Input: dimensioned drawing with shaded views. Units: mm. Origin: part minimum x, y, z. A direction names the side the tool comes from. Round coordinates to 2 decimals unless told otherwise and drop trailing zeros. Order: outer loops, then holes, each group sorted by start corner. A loop starts at its lowest first (then second) coordinate and runs counter-clockwise, first axis right, second up. Notation, with made-up numbers: M -30.75,72 L -9.75,72 A22 cw -9.75,101 Z; hole C -30.5,-12.5 d1. An arc over 180 degrees is marked long. Answer as CSV lines item,"result". Start each with the question number.
Item 1: Set-up query: the marked faces 1 and 2. Return all of +Z, -Z, +X, -X, +Y, -Y with unobstructed straight access to the full face (end or side cutting, diameter ignored); none if empty.
Item 2: Line query: line 1 (X direction, y = 23, z = 5.75); line 2 (Y direction, x = 19, z = 15.5); line 3 (Z direction, x = 17.5, y = 56.6). Output: solid intervals per line, ascending. Write a range as [from, to].
Item 3: Section query D-D on x = 32. Return the cut outline in (y, z).
Item 4: Pull-direction query (Y, two-part tool) for the marked faces 3, 4 and 5; classes: +Y half, -Y half, draft (parallel to the pull), parting line (faces both ways), or undercut.
Item 5: Section query C-C on y = 36. Return the cut outline in (x, z).
Item 6: Section query A-A on x = 17.5. Return the cut outline in (y, z), plus the area to 3 significant figures.
Item 7: Section query B-B on z = 8.25. Return the cut outline in (x, y).
Item 8: First-contact query: P1, Ø1.2, axis at x = 17.5, z = 14.56, coming from the -Y side; P2, Ø6, axis at x = 28, y = 38.5, coming from the +Z side. Flat tips, straight axial feed; report the tip coordinate or a pass-through.
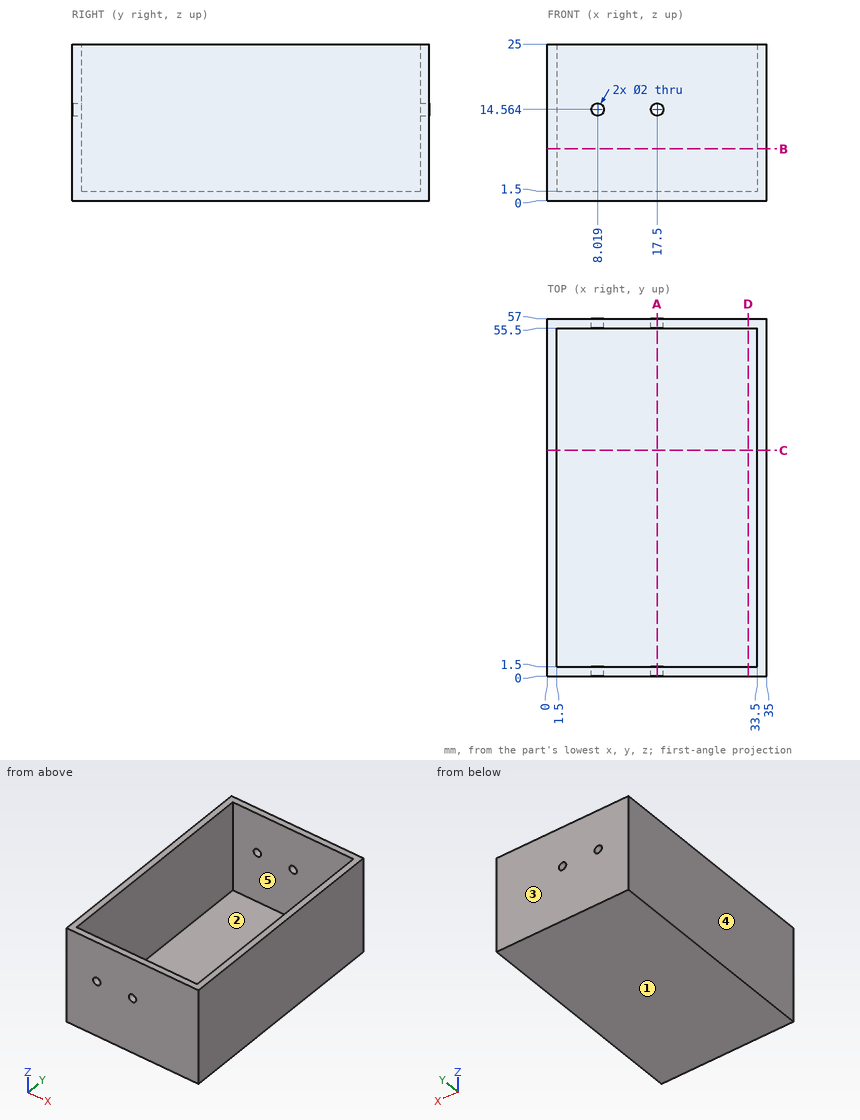
Results:
1,face 1,"-Z, +X, -X, +Y, -Y"
1,face 2,"+Z"
2,line 1,"[0, 1.5], [33.5, 35]"
2,line 2,"[0, 1.5], [55.5, 57]"
2,line 3,"[0, 13.56], [15.56, 25]"
3,outline,"M 0,0 L 57,0 L 57,25 L 55.5,25 L 55.5,1.5 L 1.5,1.5 L 1.5,25 L 0,25 Z"
4,face 3,"+Y half"
4,face 4,"draft"
4,face 5,"undercut"
5,outline,"M 0,0 L 35,0 L 35,25 L 33.5,25 L 33.5,1.5 L 1.5,1.5 L 1.5,25 L 0,25 Z"
6,outline,"M 0,0 L 57,0 L 57,13.56 L 55.5,13.56 L 55.5,1.5 L 1.5,1.5 L 1.5,13.56 L 0,13.56 Z; M 0,15.56 L 1.5,15.56 L 1.5,25 L 0,25 Z; M 55.5,15.56 L 57,15.56 L 57,25 L 55.5,25 Z"
6,area,"150 mm^2"
7,outline,"M 0,0 L 35,0 L 35,57 L 0,57 Z; hole M 1.5,1.5 L 33.5,1.5 L 33.5,55.5 L 1.5,55.5 Z"
8,P1,"through"
8,P2,"z = 1.5"
